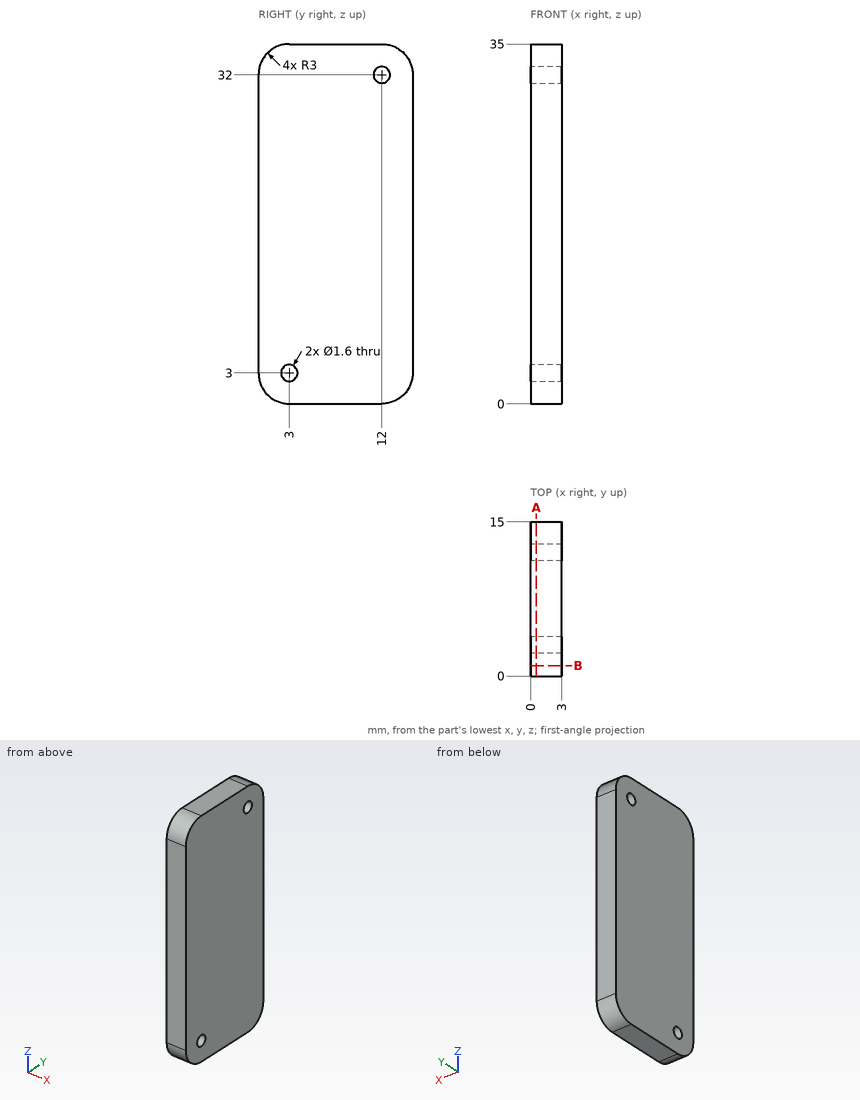
Drawing for the job (mm, zero at the part's lowest x, y, z). Round coordinates to 2 decimals unless told otherwise and drop trailing zeros. Write each loop counter-clockwise with the first axis right and the second up, starting at its lowest first coordinate (ties: lowest second). Pieces come first, ordered by that corner, then holes. Notation, with made-up numbers: (78.5, -26) - (124.5, -26) arc R17 ccw to (124.5, -12) - close; hole circle Ø7 at (86, 28). An arc over 180 degrees is marked (long way). Write item = value, one per line. Start each with the question number.
Q1. Band-saw the part on A-A (x = 0.55). Give the cut face in (y, z).
Q2. Probe L1, parallel to Y at x = 2.05, z = 32; L2, parallel to Z at x = 1.5, y = 14. List the from-to ranges inside material, lowest first. Write a range as from..to.
Q3. Band-saw the part on B-B (y = 1). Give the cut face in (x, z), then the cut area to 3 significant figures.
Answers below:
q1.outline = (0, 3) arc R3 ccw to (3, 0) - (12, 0) arc R3 ccw to (15, 3) - (15, 32) arc R3 ccw to (12, 35) - (3, 35) arc R3 ccw to (0, 32) - close; hole circle Ø1.6 at (3, 3); hole circle Ø1.6 at (12, 32)
q2.L1 = 0..11.2, 12.8..15
q2.L2 = 0.76..34.24
q3.outline = (0, 0.76) - (3, 0.76) - (3, 34.24) - (0, 34.24) - close
q3.area = 100 mm2
